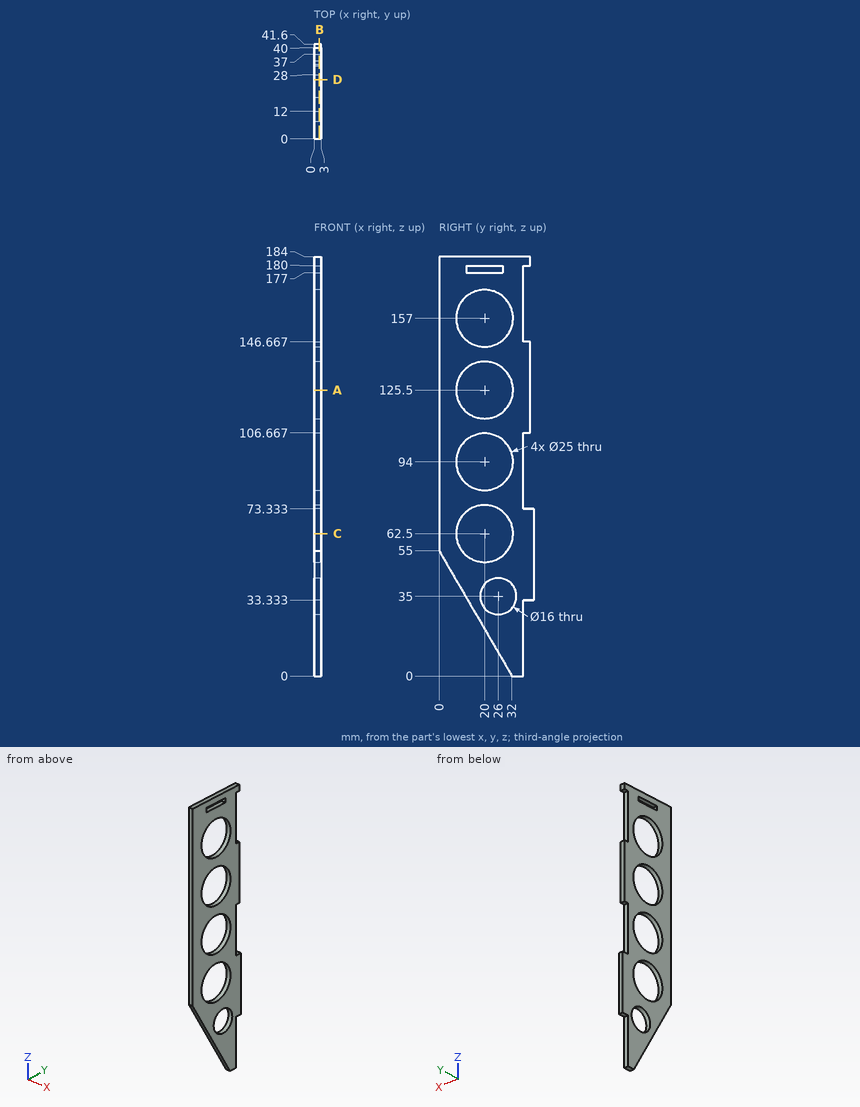
Part print with two shaded views. Sizes in mm from the minimum x, y, z corner. Give positions to 0.01 mm unless a question says otherwise; leave off trailing zeros. Order: outer loops, then holes, each group sorted by start corner. A loop starts at its lowest first (then second) coordinate and runs counter-clockwise, first axis right, second up. Notation, with made-up numbers: (45, 22.5) - (53, 22.5) arc R20 ccw to (53, 45.5) - close; hole circle Ø5 at (50, 47.25). An arc over 180 degrees is marked (long way). Write each question's results on one line, items separated by ' | '.
1. Saw through at A-A on z = 125.5. List the corners of the cut face in (x, y), and give its area (3 significant figures).
Calculated:
outline: (0, 0) - (3, 0) - (3, 7.5) - (0, 7.5) - close; (0, 32.5) - (3, 32.5) - (3, 40) - (0, 40) - close | area: 45.0 mm2
2. Probe L1, parallel to Y at x = 1.1, z = 62.5; L2, parallel to Z at x = 2.55, y = 9 (1 decimal); L3, parallel to Y at x = 1.5, z = 125.5. List the from-to ranges inside material, lowest first. Write a range as from..to.
Calculated:
L1: y = 0..7.5, 32.5..41.6 | L2: z = 39.5..56.6, 68.4..88.1, 99.9..119.6, 131.4..151.1, 162.9..184 | L3: y = 0..7.5, 32.5..40
3. Saw through at D-D on y = 26. List the corners of the cut face in (x, z), and give its area (3 significant figures).
Calculated:
outline: (0, 10.31) - (3, 10.31) - (3, 27) - (0, 27) - close; (0, 43) - (3, 43) - (3, 51.53) - (0, 51.53) - close; (0, 73.47) - (3, 73.47) - (3, 83.03) - (0, 83.03) - close; (0, 104.97) - (3, 104.97) - (3, 114.53) - (0, 114.53) - close; (0, 136.47) - (3, 136.47) - (3, 146.03) - (0, 146.03) - close; (0, 167.97) - (3, 167.97) - (3, 177) - (0, 177) - close; (0, 180) - (3, 180) - (3, 184) - (0, 184) - close | area: 201 mm2
4. Pin check, flat tips, straight feed: pin 1 (20 mm diameter, centred on y = 20, z = 125.5, fed in from -X); pin 2 (0.9 mm diameter, centred on x = 1.5, y = 40, fed in from -Z); pin 3 (0.9 mm diameter, centred on x = 2, y = 19.5, fed in from -Z); pin 4 (1 mm diameter, centred on x = 1.5, y = 15, fed in from -Z). Stop position of each tip, or through.
Calculated:
pin 1: passes through | pin 2: stops at z = 33.33 | pin 3: stops at z = 20.71 | pin 4: stops at z = 28.36
5. Saw through at B-B on x = 2.25. List the corners of the cut face in (y, z).
Calculated:
outline: (0, 55) - (32, 0) - (37, 0) - (37, 33.33) - (41.6, 33.33) - (41.6, 73.33) - (37, 73.33) - (37, 106.67) - (40, 106.67) - (40, 146.67) - (37, 146.67) - (37, 180) - (40, 180) - (40, 184) - (0, 184) - close; hole circle Ø25 at (20, 62.5); hole circle Ø25 at (20, 94); hole circle Ø25 at (20, 125.5); hole circle Ø25 at (20, 157); hole (12, 177) - (28, 177) - (28, 180) - (12, 180) - close; hole circle Ø16 at (26, 35)
6. Saw through at C-C on z = 62.5. List the corners of the cut face in (x, y).
Calculated:
outline: (0, 0) - (3, 0) - (3, 7.5) - (0, 7.5) - close; (0, 32.5) - (3, 32.5) - (3, 41.6) - (0, 41.6) - close
